Verification items for the finished model (mm, model axes). Face numbers are marked on the shaded views. Round coordinates to 2 decimals unless told otherwise and drop trailing zeros. Order: outer loops, then holes, each group sorted by start corner. A loop starts at its lowest first (then second) coordinate and runs counter-clockwise, first axis right, second up. Notation, with made-up numbers: (59, -19) -> (110, -19) arc R23 cw to (110, 18) -> close; hole circle Ø5 at (45.5, 75.25). An arc over 180 degrees is marked (long way). Return JSON: item names as keys, results as strings. Group by question number.
Item 1: Draft check along X on the marked faces 1 and 2. Enter one of: pulls with the +X half, pulls with the -X half, needs draft (parallel to the pull), parting line crosses it, or undercut.
Item 2: Sectioned sample at A-A on y = 0. Record the cut outline in (x, z).
Item 3: Depth check by flat-ended pin: pin 1 Ø3 at (y, z) = (3.5, -3) entering from -X; pin 2 Ø4 at (x, z) = (3, -3) entering from +Y; pin 3 Ø1.5 at (y, z) = (13, -1) entering from -X. Enter the tip coordinate at first touch or a pass-through.
Item 4: Sectioned sample at C-C on z = -3.25. Record the cut outline in (x, y).
Item 5: Scan lines: probe 1 along Y at (x, z) = (0, -1.9); probe 2 along X at (y, z) = (11.5, -0.5); probe 3 along Y at (x, z) = (-6.5, -4). Record each from-to range of solid material in increasing order. Write a range as from..to.
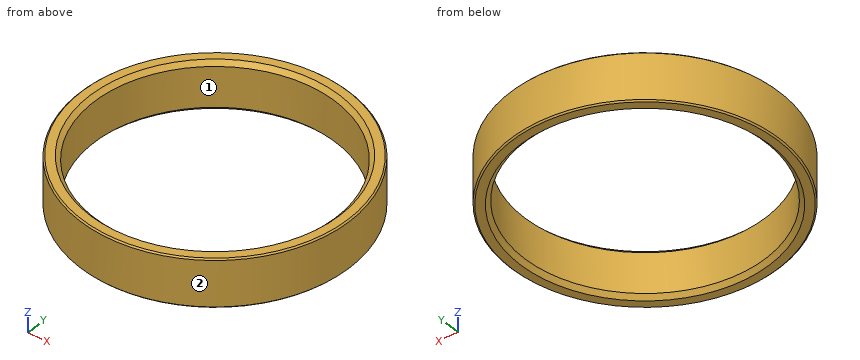
Autodesk Inventor part; units mm, degrees
ref_plane "YZ Plane" through (0, 0, 0) normal (1, 0, 0) x (0, 1, 0)
ref_plane "XZ Plane" through (0, 0, 0) normal (0, 1, 0) x (-1, 0, 0)
ref_plane "XY Plane" through (0, 0, 0) normal (0, 0, 1) x (1, 0, 0)
sketch "Sketch1" plane through (0, 0, 0) normal (0, 0, 1) x (1, 0, 0)
  circle A0 centre (0, 0) radius 19.5
  circle A1 centre (0, 0) radius 17.5
  dimension "d0" = 39
  dimension "d1" = 35
extrude "Extrusion1" add sketch "Sketch1" against normal blind 7
chamfer "Chamfer1" distance 0.6 angle 45 2 edges at (-17.5, 0, -7) (-17.5, 0, 0)
chamfer "Chamfer2" distance 0.2 angle 45 2 edges at (-19.5, 0, -7) (-19.5, 0, 0)
properties part number "6807-inner"
Recorded:
{
 "1": {"face 1": "undercut", "face 2": "parting line crosses it"},
 "2": {"outline": "(-19.5, -6.8) -> (-19.3, -7) -> (-18.1, -7) -> (-17.5, -6.4) -> (-17.5, -0.6) -> (-18.1, 0) -> (-19.3, 0) -> (-19.5, -0.2) -> close; (17.5, -6.4) -> (18.1, -7) -> (19.3, -7) -> (19.5, -6.8) -> (19.5, -0.2) -> (19.3, 0) -> (18.1, 0) -> (17.5, -0.6) -> close"},
 "3": {"pin 1": "x = -19.4", "pin 2": "y = 19.47", "pin 3": "x = -15.17"},
 "4": {"outline": "circle Ø39 at (0, 0); hole circle Ø35 at (0, 0)"},
 "5": {"probe 1": "-19.5..-17.5, 17.5..19.5", "probe 2": "-15.75..-13.32, 13.32..15.75", "probe 3": "-18.38..-16.25, 16.25..18.38"}
}
